Drawing for the job (mm, zero at the part's lowest x, y, z). Coordinates: 2 decimals unless noted, no trailing zeros. Write each loop counter-clockwise with the first axis right and the second up, starting at its lowest first coordinate (ties: lowest second). Pieces come first, ordered by that corner, then holes. Notation, with made-up numbers: M -23.75,83.5 L 15.25,83.5 A16 ccw 15.25,111.5 Z; hole C 84,-19.75 d9. An arc over 180 degrees is marked long. Use CSV: the item, a comma, the result in double quotes. Start each with the question number.
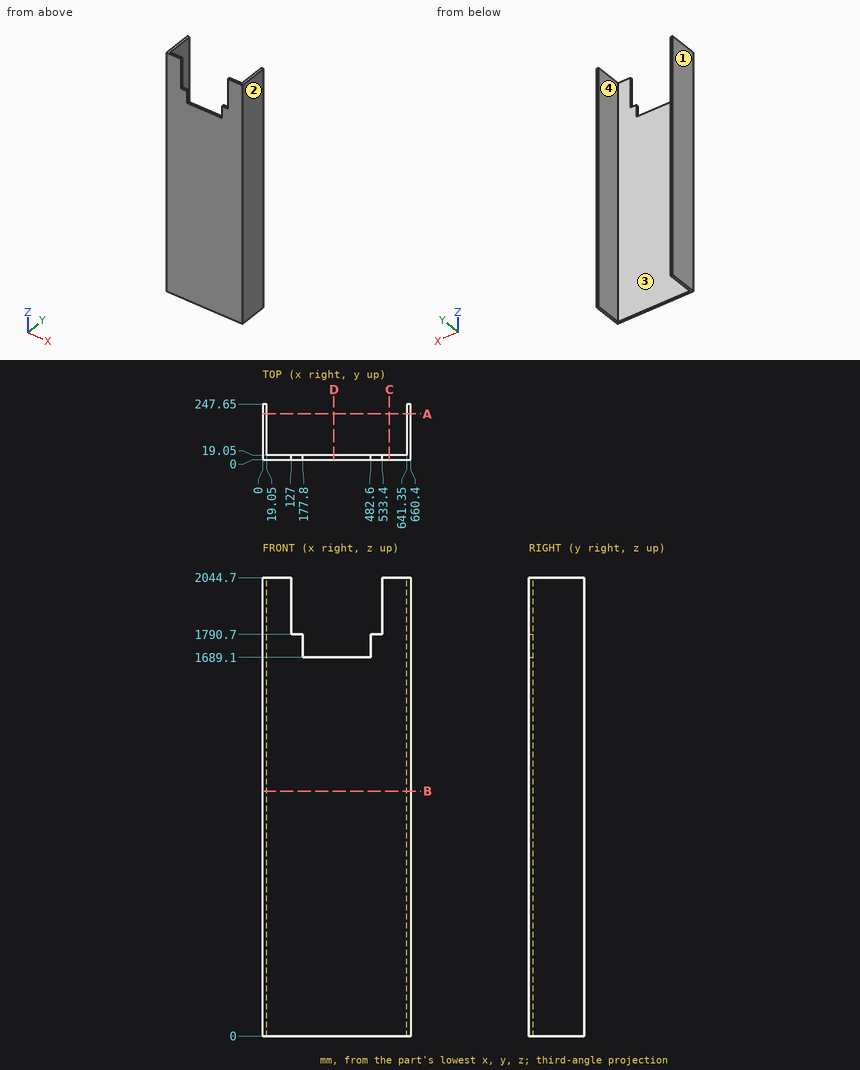
1) Band-saw the part on A-A on y = 204. List the corners of the cut face in (x, z), then the cut area to 3 significant figures.
2) Band-saw the part on D-D on x = 317.5. List the corners of the cut face in (y, z), then the cut area to 3 significant figures.
3) Band-saw the part on C-C on x = 565.5. List the corners of the cut face in (y, z).
4) Wall check: L1, parallel to X at y = 103, z = 123; L2, parallel to Y at x = 68, z = 997; L3, parallel to Z at x = 274.5, y = 18. Give the ranges that are in metal, low to high. Write a range as [from, to].
5) Two-plate mould, pull along X, no slides. Class the marked faces 1, 2, 3 and 4: pulls with the +X half, pulls with the -X half, needs draft (parallel to the pull), parting line crosses it, or undercut.
6) Band-saw the part on B-B on z = 1092. List the corners of the cut face in (x, y), then the cut area to 3 significant figures.
7) Drop flat-ended pins along their axis: P1, Ø9.5, axis at y = 14, z = 1756.5, coming from the -X side; P2, Ø1.5, axis at x = 146, z = 1150, coming from the +Y side; P3, Ø5.5, axis at x = 146, y = 10, coming from the +Z side; P4, Ø21, axis at x = 254.5, y = 12.5, coming from the +Z side. Give the stop position or say it passes through.
Findings below:
1,outline,"M 0,0 L 19.05,0 L 19.05,2044.7 L 0,2044.7 Z; M 641.35,0 L 660.4,0 L 660.4,2044.7 L 641.35,2044.7 Z"
1,area,"77,900 mm2"
2,outline,"M 0,0 L 19.05,0 L 19.05,1689.1 L 0,1689.1 Z"
2,area,"32,200 mm2"
3,outline,"M 0,0 L 19.05,0 L 19.05,2044.7 L 0,2044.7 Z"
4,L1,"x = [0, 19.05], [641.35, 660.4]"
4,L2,"y = [0, 19.05]"
4,L3,"z = [0, 1689.1]"
5,face 1,"pulls with the -X half"
5,face 2,"pulls with the +X half"
5,face 3,"undercut"
5,face 4,"undercut"
6,outline,"M 0,0 L 660.4,0 L 660.4,247.65 L 641.35,247.65 L 641.35,19.05 L 19.05,19.05 L 19.05,247.65 L 0,247.65 Z"
6,area,"21,300 mm2"
7,P1,"stops at x = 0"
7,P2,"stops at y = 19.05"
7,P3,"stops at z = 1790.7"
7,P4,"stops at z = 1689.1"
